Read the model definition and answer for the solid it produces. Units are mm, in the model's axes. Face numbers are marked on the shaded views. A direction names the side the tool comes from. Coordinates: 2 decimals unless noted, no trailing zeros. Write each loop counter-clockwise with the first axis right and the second up, starting at its lowest first coordinate (ties: lowest second). Pieces come first, ordered by that corner, then holes. Notation, with made-up numbers: (33.25, 15.25) -> (68.25, 15.25) arc R19 ccw to (68.25, 33.25) -> close; hole circle Ø10 at (18, 81). An arc over 180 degrees is marked (long way). Answer in a Markdown table with one row per item. Add a question column.
Item 1: Section A-A on x = 20 is taken. Write down the section's boundary in (y, z), then the cut area to 3 significant figures.
Item 2: Which of the six approach directions +Z, -Z, +X, -X, +Y, -Y give full straight-line access (tool end or side, diameter ignored) to the marked faces 1 and 2?
Item 3: Straight lines are drawn through the part: line 1 (Y direction, x = 51, z = -14); line 2 (X direction, y = 8, z = -5.5); line 3 (Z direction, x = 14.5, y = 8). For each, find the intervals that lie inside material, in ascending order. Write a range as from..to.
Item 4: Section D-D on y = 8 is taken. Write down the section's boundary in (x, z), then the cut area to 3 significant figures.
Item 5: Section B-B on y = 5 is taken. Write down the section's boundary in (x, z).
Item 6: Given pin 1 Ø1.2 at (x, y) = (37.5, 5) entering from +Z; pin 2 Ø10 at (x, z) = (18, -12) entering from +Y; pin 3 Ø0.6 at (y, z) = (8.5, -9) entering from +X, each flat-ended and moving along its own axis, determine where each tip first touches the part or whether it passes through.
Item 7: Section C-C on z = -21.5 is taken. Write down the section's boundary in (x, y).
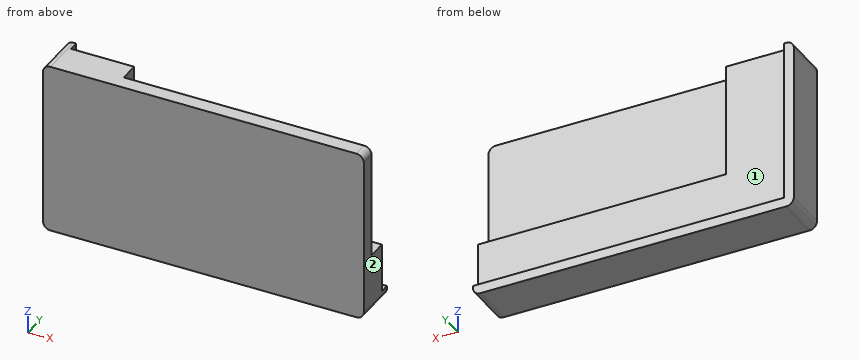
```python
from build123d import *

# Parameters (mm, degrees)
SKETCH1_W           = 65
SKETCH1_H           = 35
BOSS_EXTRUDE1_DEPTH = 9
SKETCH2_W           = 63
SKETCH2_H           = 33
CUT_EXTRUDE1_DEPTH  = 2
SKETCH3_W           = 50.2
SKETCH3_H           = 23
CUT_EXTRUDE2_DEPTH  = 4
FILLET1_R           = 1.5


with BuildPart() as part:
    # Sketch1 → Boss-Extrude1 (new body)
    with BuildSketch(Plane(origin=(0, 0, 0), x_dir=(1, 0, 0), z_dir=(0, 1, 0))):
        with Locations((32.5, 17.5)):
            Rectangle(SKETCH1_W, SKETCH1_H)
    extrude(amount=BOSS_EXTRUDE1_DEPTH)

    # Sketch2 → Cut-Extrude1 (cut)
    with BuildSketch(Plane(origin=(0, 9, 0), x_dir=(1, 0, 0), z_dir=(0, 1, 0))):
        with Locations((33.5, 16.5)):
            Rectangle(SKETCH2_W, SKETCH2_H)
    extrude(amount=-CUT_EXTRUDE1_DEPTH, mode=Mode.SUBTRACT)

    # Sketch3 → Cut-Extrude2 (cut)
    with BuildSketch(Plane(origin=(0, 7, 0), x_dir=(1, 0, 0), z_dir=(0, 1, 0))):
        with Locations((39.9, 11.5)):
            Rectangle(SKETCH3_W, SKETCH3_H)
    extrude(amount=-CUT_EXTRUDE2_DEPTH, mode=Mode.SUBTRACT)

    # Fillet1
    fillet1_edges = [part.edges().sort_by_distance(p)[0] for p in [
        (65, 1.5, 0),
        (0, 4.5, -35),
        (65, 4.5, -35),
        (0, 4.5, 0),
    ]]
    fillet(fillet1_edges, radius=FILLET1_R)


solid = part.part
```
Results below:
| question | item | result |
|---|---|---|
| 1 | outline | (0, -35) -> (9, -35) -> (9, -33) -> (7, -33) -> (7, -23) -> (3, -23) -> (3, 0) -> (0, 0) -> close |
| 1 | area | 157 mm2 |
| 2 | face 1 | +Z, +X, +Y |
| 2 | face 2 | +Z, -Z, +X, +Y, -Y |
| 3 | line 1 | y = 0..3 |
| 3 | line 2 | x = 0..2 |
| 3 | line 3 | z = -35..-33 |
| 4 | outline | (0, -33.5) arc R1.5 ccw to (1.5, -35) -> (63.5, -35) arc R1.5 ccw to (65, -33.5) -> (65, -33) -> (2, -33) -> (2, 0) -> (1.5, 0) arc R1.5 ccw to (0, -1.5) -> close |
| 4 | area | 195 mm2 |
| 5 | outline | (0, -33.5) arc R1.5 ccw to (1.5, -35) -> (63.5, -35) arc R1.5 ccw to (65, -33.5) -> (65, -23) -> (14.8, -23) -> (14.8, 0) -> (1.5, 0) arc R1.5 ccw to (0, -1.5) -> close |
| 6 | pin 1 | stops at z = -23 |
| 6 | pin 2 | stops at y = 7 |
| 6 | pin 3 | stops at x = 2 |
| 7 | outline | (0, 0) -> (65, 0) -> (65, 3) -> (14.8, 3) -> (14.8, 7) -> (2, 7) -> (2, 9) -> (0, 9) -> close |
